Design review of the part built by this model. Coordinates are the model's own, in mm. Coordinates: 2 decimals unless noted, no trailing zeros. Write each loop counter-clockwise with the first axis right and the second up, starting at its lowest first coordinate (ties: lowest second). Pieces come first, ordered by that corner, then holes. Notation, with made-up numbers: M 18,13 L 53,13 A16 ccw 53,33 Z; hole C 87,-8.5 d9. An arc over 180 degrees is marked long. One line per question, with ' | ' between items.
from build123d import *

# Parameters (mm, degrees)
SKETCH1_R              = 12.5
BOSS_EXTRUDE1_DEPTH    = 35
BOSS_EXTRUDE1_TAPER    = -45
SKETCH2_R              = 7.5
SUPPORT_ARM_HOLE_DEPTH = 71.0000001


with BuildPart() as part:
    # Sketch1 → Boss-Extrude1 (new body)
    with BuildSketch(Plane(origin=(0, 0, 0), x_dir=(0, 0, -1), z_dir=(1, 0, 0))):
        Circle(SKETCH1_R)
    boss_extrude1 = extrude(amount=BOSS_EXTRUDE1_DEPTH, taper=BOSS_EXTRUDE1_TAPER)

    # Mirror1: Boss-Extrude1 across plane
    add(boss_extrude1.mirror(Plane(origin=(0, 0, 0), x_dir=(0, 0, 1), z_dir=(1, 0, 0))))

    # Sketch2 → Support Arm Hole (cut, through all)
    with BuildSketch(Plane(origin=(35, 0, 0), x_dir=(0, 0, -1), z_dir=(1, 0, 0))):
        Circle(SKETCH2_R)
    extrude(amount=-SUPPORT_ARM_HOLE_DEPTH, mode=Mode.SUBTRACT)


solid = part.part
1. To check wall thickness, follow line 1 along Z through (x, y) = (11.5, -5.5); line 2 along X through (y, z) = (-23.5, 10); line 3 along Y through (x, z) = (-28, 3). State the ranges of each line that lie inside material, in increasing order. Write a range as [from, to].
Answer sheet:
line 1: [-23.36, -5.1], [5.1, 23.36] | line 2: [-35, -13.04], [13.04, 35] | line 3: [-40.39, -6.87], [6.87, 40.39]
2. Draft analysis for pull direction X (two halves, no side actions). For faces 1 (the face through (0.49, 0.33, 7.493)), 2 (the face through (-35, 1, -10)), 3 (the face through (-2.19, -14.34, 3.18)), 4 (the face through (35, 1, -10)), state which applies: pulls with the +X half, pulls with the -X half, needs draft (parallel to the pull), parting line crosses it, or undercut.
Answer sheet:
face 1: needs draft | face 2: pulls with the -X half | face 3: undercut | face 4: pulls with the +X half
3. Take a section at B-B (x = 23.5). Write out the cut boundary in (y, z), then the cut area to 3 significant figures.
Answer sheet:
outline: C 0,0 d72; hole C 0,0 d15 | area: 3,890 mm^2
4. Take a section at A-A (z = 0). Write out the cut boundary in (x, y).
Answer sheet:
outline: M -35,-47.5 L 0,-12.5 L 35,-47.5 L 35,-7.5 L -35,-7.5 Z; M -35,7.5 L 35,7.5 L 35,47.5 L 0,12.5 L -35,47.5 Z
5. Take a section at C-C (x = -9). Write out the cut boundary in (y, z), then the cut area to 3 significant figures.
Answer sheet:
outline: C 0,0 d43; hole C 0,0 d15 | area: 1,280 mm^2
6. Insertion check: pin 1 Ø9 at (y, z) = (0, 0) entering from +X; pin 2 Ø4 at (x, y) = (-24.5, -9.5) entering from +Z; pin 3 Ø4 at (x, z) = (-9.5, 17) entering from -Y. Each pin has a flat end and moves straight along its axis. Give the tip position at first contact, or say it passes through.
Answer sheet:
pin 1: through | pin 2: z = 37.88 | pin 3: y = -17.54
